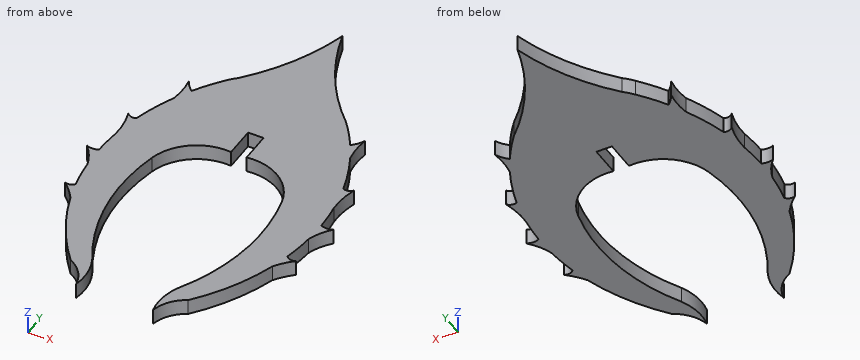
from build123d import *

# Parameters (mm, degrees)
BOSS_EXTRUDE1_DEPTH = 1.524


with BuildPart() as part:
    # Sketch1 → Boss-Extrude1 (new body)
    with BuildSketch(Plane.XY):
        with BuildLine():
            Line((-0.760070899, 7.460977954), (0.767897128, 7.459984541))
            Line((0.767897128, 7.459984541), (0.765910301, 4.411002891))
            ThreePointArc((0.765910301, 4.411002891), (4.32194984, 3.493667889), (6.372371333, 0.446916765))
            ThreePointArc((6.372371333, 0.446916765), (6.688594723, -7.066471539), (4.226511646, -14.172043153))
            ThreePointArc((4.226511646, -14.172043153), (3.666960455, -16.006802716), (3.76324428, -17.922571391))
            ThreePointArc((3.76324428, -17.922571391), (4.445796565, -16.344729964), (5.770776644, -15.249335522))
            ThreePointArc((5.770776644, -15.249335522), (8.209412547, -11.678891072), (9.901915798, -7.700141093))
            ThreePointArc((9.901915798, -7.700141093), (10.56591512, -6.836092284), (11.345730748, -6.07493328))
            ThreePointArc((11.345730748, -6.07493328), (10.826887202, -6.157946188), (10.391178227, -5.864267011))
            ThreePointArc((10.391178227, -5.864267011), (10.661740328, -4.406185462), (10.833367262, -2.933178384))
            ThreePointArc((10.833367262, -2.933178384), (11.345730748, -1.758358454), (12.109295167, -0.728947171))
            ThreePointArc((12.109295167, -0.728947171), (11.509245819, -0.877984338), (10.904429696, -0.749653693))
            ThreePointArc((10.904429696, -0.749653693), (10.842155911, 0.568514134), (10.700889839, 1.880569141))
            ThreePointArc((10.700889839, 1.880569141), (10.750460558, 3.375199082), (11.072247287, 4.835619986))
            ThreePointArc((11.072247287, 4.835619986), (10.654347315, 4.554276024), (10.151679138, 4.587735186))
            ThreePointArc((10.151679138, 4.587735186), (9.493497129, 6.629427415), (8.639426453, 8.597236857))
            ThreePointArc((8.639426453, 8.597236857), (8.516035962, 9.943618933), (8.639426453, 11.29000101))
            ThreePointArc((8.639426453, 11.29000101), (8.278476637, 10.67654613), (7.787243967, 10.161471258))
            ThreePointArc((7.787243967, 10.161471258), (6.925869801, 11.489539462), (5.971147131, 12.752169745))
            ThreePointArc((5.971147131, 12.752169745), (2.303316115, 17.492889529), (0.004783201, 23.028605823))
            ThreePointArc((0.004783201, 23.028605823), (-1.992221452, 18.030222496), (-5.110354293, 13.642841609))
            ThreePointArc((-5.110354293, 13.642841609), (-5.554708445, 13.214619989), (-5.963320902, 12.752169745))
            ThreePointArc((-5.963320902, 12.752169745), (-6.918043572, 11.489539462), (-7.779417738, 10.161471258))
            ThreePointArc((-7.779417738, 10.161471258), (-8.270650408, 10.67654613), (-8.631600224, 11.29000101))
            ThreePointArc((-8.631600224, 11.29000101), (-8.508209733, 9.943618933), (-8.631600224, 8.597236857))
            ThreePointArc((-8.631600224, 8.597236857), (-9.4856709, 6.629427415), (-10.14385291, 4.587735186))
            ThreePointArc((-10.14385291, 4.587735186), (-10.646521087, 4.554276024), (-11.064421059, 4.835619986))
            ThreePointArc((-11.064421059, 4.835619986), (-10.742634329, 3.375199082), (-10.69306361, 1.880569141))
            ThreePointArc((-10.69306361, 1.880569141), (-10.834329682, 0.568514134), (-10.896603467, -0.749653693))
            ThreePointArc((-10.896603467, -0.749653693), (-11.50141959, -0.877984338), (-12.101468938, -0.728947171))
            ThreePointArc((-12.101468938, -0.728947171), (-11.33790452, -1.758358454), (-10.825541034, -2.933178384))
            ThreePointArc((-10.825541034, -2.933178384), (-10.653914099, -4.406185462), (-10.383351998, -5.864267011))
            ThreePointArc((-10.383351998, -5.864267011), (-10.819060973, -6.157946188), (-11.33790452, -6.07493328))
            ThreePointArc((-11.33790452, -6.07493328), (-10.558088891, -6.836092284), (-9.894089569, -7.700141093))
            ThreePointArc((-9.894089569, -7.700141093), (-8.201586318, -11.678891072), (-5.762950415, -15.249335522))
            ThreePointArc((-5.762950415, -15.249335522), (-4.437970336, -16.344729964), (-3.755418051, -17.922571391))
            ThreePointArc((-3.755418051, -17.922571391), (-3.659134226, -16.006802716), (-4.218685417, -14.172043153))
            ThreePointArc((-4.218685417, -14.172043153), (-6.680768494, -7.066471539), (-6.364545104, 0.446916765))
            ThreePointArc((-6.364545104, 0.446916765), (-4.314549444, 3.493366768), (-0.759120805, 4.411117837))
            Line((-0.759120805, 4.411117837), (-0.760070899, 7.460977954))
        make_face()
    extrude(amount=BOSS_EXTRUDE1_DEPTH)


solid = part.part
Geometry: final body of the model. Coordinates: model frame, mm. Round coordinates to 2 decimals unless told otherwise and drop trailing zeros. Order: outer loops, then holes, each group sorted by start corner. A loop starts at its lowest first (then second) coordinate and runs counter-clockwise, first axis right, second up. Notation, with made-up numbers: (-34, -38) - (-6, -38) arc R17 ccw to (-6, -6) - close; hole circle Ø4 at (47.25, 62.25). An arc over 180 degrees is marked (long way). Write each question's results on one line, items separated by ' | '.
Item 1: Section B-B, the plane y = -8.5. Return the cut outline in (x, z), and give its area (3 significant figures).
Completed:
outline: (-9.63, 0) - (-6.42, 0) - (-6.42, 1.52) - (-9.63, 1.52) - close; (6.42, 0) - (9.63, 0) - (9.63, 1.52) - (6.42, 1.52) - close | area: 9.78 mm^2
Item 2: Section D-D, the plane y = 18.5. Return the cut outline in (x, z), and give its area (3 significant figures).
Completed:
outline: (-1.74, 0) - (1.75, 0) - (1.75, 1.52) - (-1.74, 1.52) - close | area: 5.33 mm^2
Item 3: Section C-C, the plane x = -9.25. Return the cut outline in (y, z).
Completed:
outline: (-9.48, 0) - (7.23, 0) - (7.23, 1.52) - (-9.48, 1.52) - close
Item 4: Section A-A, the plane y = -2. Return the cut outline in (x, z), and give its area (3 significant figures).
Completed:
outline: (-11.21, 0) - (-6.78, 0) - (-6.78, 1.52) - (-11.21, 1.52) - close; (6.79, 0) - (11.21, 0) - (11.21, 1.52) - (6.79, 1.52) - close | area: 13.5 mm^2
Item 5: First-contact query: pin 1 Ø0.8 at (y, z) = (5.5, 1) entering from +X; pin 2 Ø1 at (x, y) = (3.5, 13) entering from -Z. Flat tips, straight axial feed; report the tip coordinate or a pass-through.
Completed:
pin 1: x = 10.01 | pin 2: z = 0
Item 6: Material intervals for line 1 along X through (y, z) = (-10, 1.2); line 2 along Y through (x, z) = (-5, 1.05); line 3 along X through (y, z) = (-14, 1.4), sorted ascending. Write a range as [from, to].
Completed:
line 1: [-9.03, -6.02], [6.03, 9.04] | line 2: [-15.75, -12.67], [2.91, 13.77] | line 3: [-6.74, -4.32], [4.32, 6.74]
